CAD build for the part. Positions are in the model's coordinates, mm. Face numbers are marked on the shaded views. A direction names the side the tool comes from. Round coordinates to 2 decimals unless told otherwise and drop trailing zeros. Write each loop counter-clockwise with the first axis right and the second up, starting at its lowest first coordinate (ties: lowest second). Pieces come first, ordered by that corner, then holes. Notation, with made-up numbers: (17.5, 87) - (34.5, 87) arc R26 ccw to (34.5, 113) - close; hole circle Ø9 at (15.5, 53). An arc over 180 degrees is marked (long way). Answer in a Markdown table with one row per item.
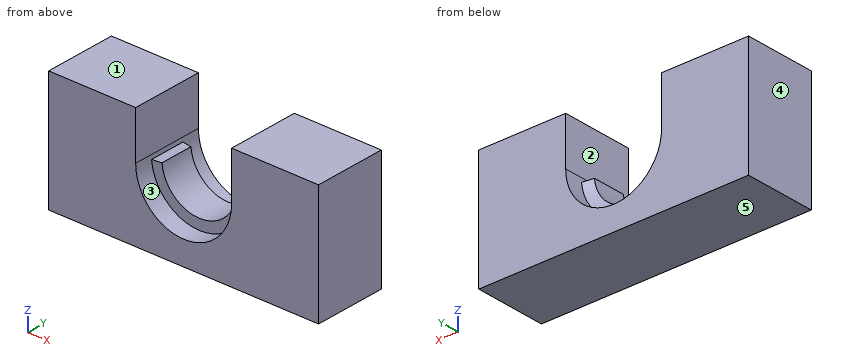
```python
from build123d import *

# Parameters (mm, degrees)
F0_W          = 45
F0_H          = 12
F1_DEPTH      = 20
F3_DEPTH      = 12.001
F5_ANGLE_BACK = 85
F5_ANGLE      = 170


with BuildPart() as f1:
    # F0 (on Top) → F1 (new body)
    with BuildSketch(Plane.XY):
        with Locations((0, 6)):
            Rectangle(F0_W, F0_H)
    extrude(amount=F1_DEPTH)

    # F2 (on face) → F3 (cut, through all)
    with BuildSketch(Plane(origin=(0, 12, 0), x_dir=(-1, 0, 0), z_dir=(0, 1, 0))):
        with BuildLine():
            ThreePointArc((-8, 12), (0, 4), (8, 12))
            Line((8, 12), (8, 20))
            Line((8, 20), (-8, 20))
            Line((-8, 20), (-8, 12))
        make_face()
    extrude(amount=-F3_DEPTH, mode=Mode.SUBTRACT)

    # F4 (on Right) → F5 (revolve)
    with BuildSketch(Plane.YZ, mode=Mode.PRIVATE) as f5_sk:
        Polygon((3, 4), (9, 4), (8.5310889132, 5.75), (3, 5.75), align=None)
    revolve(f5_sk.sketch.rotate(Axis((0, 6, 12), (0, -1, 0)), -F5_ANGLE_BACK), axis=Axis((0, 6, 12), (0, -1, 0)), revolution_arc=F5_ANGLE)


solid = f1.part
```
Q1. Saw through at C-C on y = 1.25. List the corners of the cut face in (x, z).
Computed:
| item | result |
|---|---|
| outline | (-22.5, 0) - (22.5, 0) - (22.5, 20) - (8, 20) - (8, 12) arc R8 cw to (-8, 12) - (-8, 20) - (-22.5, 20) - close |
Q2. Saw through at B-B on x = 0. List the corners of the cut face in (y, z).
Computed:
| item | result |
|---|---|
| outline | (0, 0) - (12, 0) - (12, 4) - (9, 4) - (8.53, 5.75) - (3, 5.75) - (3, 4) - (0, 4) - close |
Q3. Saw through at D-D on y = 6.5. List the corners of the cut face in (x, z).
Computed:
| item | result |
|---|---|
| outline | (-22.5, 0) - (22.5, 0) - (22.5, 20) - (8, 20) - (8, 12) arc R8 cw to (7.97, 11.3) - (6.23, 11.46) arc R6.25 cw to (-6.23, 11.46) - (-7.97, 11.3) arc R8 cw to (-8, 12) - (-8, 20) - (-22.5, 20) - close |
Q4. Pull direction X, two halves, no side cores. Call the marked faces 3, 4 and 5: released by +X, released by -X, zero draft, split by the parting line, or undercut.
Computed:
| item | result |
|---|---|
| face 3 | undercut |
| face 4 | released by -X |
| face 5 | zero draft |
Q5. 3-axis set-ups, long thin cutter, end or side, ignore diameter. For the marked faces 1 and 2: which of +Z, -Z, +X, -X, +Y, -Y reach the whole face in a straight line?
Computed:
| item | result |
|---|---|
| face 1 | +Z, +X, -X, +Y, -Y |
| face 2 | +Z, +Y, -Y |
Q6. Drill centre lines: line 1 (X direction, y = 8, z = 16.25); line 2 (Z direction, x = 5, y = 10) (3 decimals); line 3 (X direction, y = 11.75, z = 7.25). Where is each one in solid material? Low to high.
Computed:
| item | result |
|---|---|
| line 1 | x = -22.5 to -8, 8 to 22.5 |
| line 2 | z = 0 to 5.755 |
| line 3 | x = -22.5 to -6.44, 6.44 to 22.5 |
Q7. Flat gauge pin, fed straight in: pin 1 (3.5 mm diameter, centred on x = 0, z = 7, fed in from -Y). Where does the tip first touch, or does it go through?
Computed:
| item | result |
|---|---|
| pin 1 | stops at y = 3 |
Q8. Saw through at A-A on z = 15.75. List the corners of the cut face in (x, y), then the cut area to 3 significant figures.
Computed:
| item | result |
|---|---|
| outline | (-22.5, 0) - (-8, 0) - (-8, 12) - (-22.5, 12) - close; (8, 0) - (22.5, 0) - (22.5, 12) - (8, 12) - close |
| area | 348 mm2 |
